Print and shaded views of the part. All mm, measured from the part's lowest x, y and z. A direction names the side the tool comes from. Round coordinates to 2 decimals unless told otherwise and drop trailing zeros. Loops run counter-clockwise (first coordinate to the right, second up) from the corner with the lowest first, then second, coordinate; pieces in that order, holes last. Notation, with made-up numbers: (89.25, 27.5) -> (106.25, 27.5) arc R23 ccw to (106.25, 43.5) -> close; hole circle Ø10 at (23, 51). An arc over 180 degrees is marked (long way). Answer as CSV lines item,"result".
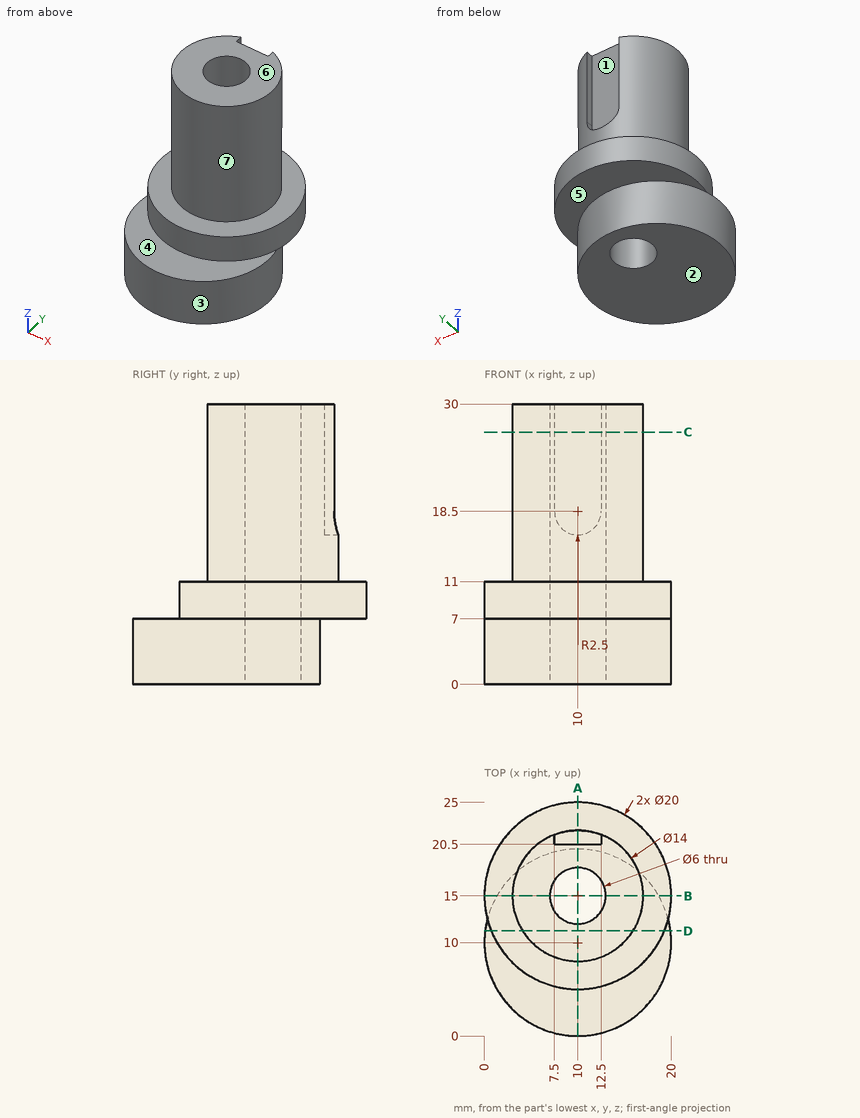
Q1. Two-plate mould, pull along X, no slides. Class the marked faces 1, 2 and 3: pulls with the +X half, pulls with the -X half, needs draft (parallel to the pull), parting line crosses it, or undercut.
Results:
face 1,"undercut"
face 2,"needs draft"
face 3,"parting line crosses it"
Q2. Probe L1, parallel to Y at x = 10, z = 13.5; L2, parallel to Y at x = 10, z = 20.25; L3, parallel to Z at x = 4.5, y = 22. List the from-to ranges inside material, lowest first. Write a range as [from, to].
Results:
L1,"[8, 12], [18, 22]"
L2,"[8, 12], [18, 20.5]"
L3,"[7, 11]"
Q3. Slice it at A-A, the plane x = 10. Give the cut face in (y, z), and give its area (3 significant figures).
Results:
outline,"(0, 0) -> (12, 0) -> (12, 30) -> (8, 30) -> (8, 11) -> (5, 11) -> (5, 7) -> (0, 7) -> close; (18, 0) -> (20, 0) -> (20, 7) -> (25, 7) -> (25, 11) -> (22, 11) -> (22, 16) -> (20.5, 16) -> (20.5, 30) -> (18, 30) -> close"
area,"285 mm2"
Q4. Drop flat-ended pins along their axis: pin 1 Ø2.5 at (x, z) = (9, 20.5) entering from +Y; pin 2 Ø10 at (y, z) = (6.5, 21) entering from -X; pin 3 Ø10 at (x, z) = (7, 20) entering from -Y; pin 4 Ø5.5 at (x, y) = (10, 15) entering from +Z. Give the stop position or say it passes through.
Results:
pin 1,"y = 20.5"
pin 2,"x = 3.94"
pin 3,"y = 8"
pin 4,"through"
Q5. Slice it at B-B, the plane y = 15. Give the cut face in (x, z), and give its area (3 significant figures).
Results:
outline,"(0, 7) -> (1.34, 7) -> (1.34, 0) -> (7, 0) -> (7, 30) -> (3, 30) -> (3, 11) -> (0, 11) -> close; (13, 0) -> (18.66, 0) -> (18.66, 7) -> (20, 7) -> (20, 11) -> (17, 11) -> (17, 30) -> (13, 30) -> close"
area,"287 mm2"
Q6. Tool access for the marked faces 4, 5, 6 and 7: list every direction of +Z, -Z, +X, -X, +Y, -Y with a clear straight run to the whole face (end or side of a thin tool).
Results:
face 4,"+Z, -Y"
face 5,"-Z, +Y"
face 6,"+Z, +X, -X, +Y, -Y"
face 7,"+Z"
Q7. Slice it at D-D, the plane y = 11.25. Give the cut face in (x, z).
Results:
outline,"(0.08, 0) -> (19.92, 0) -> (19.92, 7) -> (19.27, 7) -> (19.27, 11) -> (15.91, 11) -> (15.91, 30) -> (4.09, 30) -> (4.09, 11) -> (0.73, 11) -> (0.73, 7) -> (0.08, 7) -> close"
Q8. Slice it at C-C, the plane z = 27. Give the cut face in (x, y), and give its area (3 significant figures).
Results:
outline,"(7.5, 20.5) -> (7.5, 21.54) arc R7 ccw (long way) to (12.5, 21.54) -> (12.5, 20.5) -> close; hole circle Ø6 at (10, 15)"
area,"119 mm2"
